from build123d import *

# Parameters (mm, degrees)
SKETCH28_W                                   = 80
SKETCH28_H                                   = 80
BOSS_EXTRUDE1_DEPTH                          = 10
CBORE_FOR_M10_CHEESE_HEAD_SCREW1_D           = 12
CBORE_FOR_M10_CHEESE_HEAD_SCREW1_CBORE_D     = 26
CBORE_FOR_M10_CHEESE_HEAD_SCREW1_CBORE_DEPTH = 5
SKETCH36_R                                   = 1
BOSS_EXTRUDE5_DEPTH                          = 10
SKETCH37_R                                   = 22.5
SKETCH37_R_2                                 = 15.5
CUT_EXTRUDE2_DEPTH                           = 6
CUT_EXTRUDE6_DEPTH                           = 6
SKETCH40_W                                   = 18.062589032
SKETCH40_H                                   = 3
BOSS_EXTRUDE7_DEPTH                          = 13


with BuildPart() as part:
    # Sketch28 → Boss-Extrude1 (new body)
    with BuildSketch(Plane(origin=(0, 0, 0), x_dir=(1, 0, 0), z_dir=(0, 1, 0))):
        with Locations((1.944585414, 4.241283073)):
            Rectangle(SKETCH28_W, SKETCH28_H)
    extrude(amount=BOSS_EXTRUDE1_DEPTH)

    # CBORE for M10 Cheese Head Screw1 (through all)
    with Locations(Plane(origin=(0, 10, 0), x_dir=(1, 0, 0), z_dir=(0, 1, 0))):
        with Locations((1.944585414, 4.241283073)):
            CounterBoreHole(CBORE_FOR_M10_CHEESE_HEAD_SCREW1_D / 2, CBORE_FOR_M10_CHEESE_HEAD_SCREW1_CBORE_D / 2, CBORE_FOR_M10_CHEESE_HEAD_SCREW1_CBORE_DEPTH)

    # Sketch36 → Boss-Extrude5 (add)
    with BuildSketch(Plane.XZ):
        with Locations(Location((12.444585414, -16.741283073, 0), (0, 0, 270))):
            Circle(SKETCH36_R)
        with Locations(Location((12.444585414, -4.241283073, 0), (0, 0, 270))):
            Circle(SKETCH36_R)
        with Locations(Location((-8.555414586, -16.741283073, 0), (0, 0, 90))):
            Circle(SKETCH36_R)
        with Locations(Location((-8.555414586, -4.241283073, 0), (0, 0, 90))):
            Circle(SKETCH36_R)
    extrude(amount=BOSS_EXTRUDE5_DEPTH)

    # Sketch37 → Cut-Extrude2 (cut)
    with BuildSketch(Plane(origin=(0, 10, 0), x_dir=(1, 0, 0), z_dir=(0, 1, 0))):
        with Locations(Location((1.944585414, 4.241283073, 0), (0, 0, 270))):
            Circle(SKETCH37_R)
        with Locations(Location((1.944585414, 4.241283073, 0), (0, 0, 270))):
            Circle(SKETCH37_R_2, mode=Mode.SUBTRACT)
    extrude(amount=-CUT_EXTRUDE2_DEPTH, mode=Mode.SUBTRACT)

    # Sketch39 → Cut-Extrude6 (cut)
    with BuildSketch(Plane(origin=(0, 10, 0), x_dir=(1, 0, 0), z_dir=(0, 1, 0))):
        with BuildLine():
            Line((6.944585414, -35.758716927), (6.944585414, -17.696127895))
            ThreePointArc((6.944585414, -17.696127895), (1.944585414, -18.258716927), (-3.055414586, -17.696127895))
            Line((-3.055414586, -17.696127895), (-3.055414586, -35.758716927))
            Line((-3.055414586, -35.758716927), (1.944585414, -35.758716927))
            Line((1.944585414, -35.758716927), (6.944585414, -35.758716927))
        make_face()
    extrude(amount=-CUT_EXTRUDE6_DEPTH, mode=Mode.SUBTRACT)

    # Sketch40 → Boss-Extrude7 (add)
    with BuildSketch(Plane(origin=(-3.055414586, 0, 0), x_dir=(0, 0, -1), z_dir=(1, 0, 0))):
        with Locations((-26.727422411, 8.5)):
            Rectangle(SKETCH40_W, SKETCH40_H)
    extrude(amount=BOSS_EXTRUDE7_DEPTH)


solid = part.part
Geometry check sheet. Reference: the model listing, model coordinates, mm. A direction names the side the tool comes from. Coordinates: 2 decimals unless noted, no trailing zeros. Order: outer loops, then holes, each group sorted by start corner. A loop starts at its lowest first (then second) coordinate and runs counter-clockwise, first axis right, second up. Notation, with made-up numbers: (30, 8) -> (61, 8) arc R19 ccw to (61, 25) -> close; hole circle Ø8 at (-1.75, 9.5). An arc over 180 degrees is marked (long way). Use a Markdown table: item, result. Add a question column.
1. Cross-section at A-A (z = 0). Enter the section's corners in (x, y).
2. Go/stop test with flat-tipped pins: pin 1 Ø24 at (x, z) = (12, 14.5) entering from -Y; pin 2 Ø13 at (x, z) = (5, -5) entering from +Y; pin 3 Ø23.5 at (x, z) = (1.94, -4.24) entering from -Y. Record where each tip stops, or that it passes through.
3. Cross-section at D-D (y = -4.25). Enter the section's corners in (x, z).
4. Mould release check, pull along X, two halves, no side actions. Record for faces 1 (the face through (2.863, 7.042, -26.723)), 2 (the face through (7.94, 2.46, -4.51)), 3 (the face through (-9, -10, -17)), 4 (the face through (-38.055, 5, -4)): pulls with the +X half, pulls with the -X half, needs draft (parallel to the pull), parting line crosses it, or undercut.
5. Set-up check for faces 5 (the face through (1, 5, -44.241)), 6 (the face through (11.557, -4.93, -4.703)), 7 (the face through (-0.87, 7.54, 8.45)), 8 (the face through (-16, 10, -21)), 9 (the face through (2, 7, 27)): record each of +Z, -Z, +X, -X, +Y, -Y from which the full face is reachable in a straight line by a thin tool's end or side.
6. Cross-section at B-B (z = 27). Enter the section's corners in (x, y).
7. Cross-section at C-C (x = -24). Enter the section's corners in (y, z), and give its area (3 significant figures).
8. Material ranges on L1, parallel to X at y = 5, z = 26; L2, parallel to Z at x = 10, y = 4.5; L3, parallel to X at y = 8.75, z = -12.5, recorded low to high.
Filled sheet:
| question | item | result |
|---|---|---|
| 1 | outline | (-38.06, 0) -> (-2.3, 0) -> (-2.3, 5) -> (-10.34, 5) -> (-10.34, 10) -> (-12.96, 10) -> (-12.96, 4) -> (-20.15, 4) -> (-20.15, 10) -> (-38.06, 10) -> close; (6.19, 0) -> (41.94, 0) -> (41.94, 10) -> (24.04, 10) -> (24.04, 4) -> (16.85, 4) -> (16.85, 10) -> (14.23, 10) -> (14.23, 5) -> (6.19, 5) -> close |
| 2 | pin 1 | y = 0 |
| 2 | pin 2 | y = 5 |
| 2 | pin 3 | y = -10 |
| 3 | outline | circle Ø2 at (-8.56, -16.74); circle Ø2 at (-8.56, -4.24); circle Ø2 at (12.44, -16.74); circle Ø2 at (12.44, -4.24) |
| 4 | face 1 | undercut |
| 4 | face 2 | undercut |
| 4 | face 3 | needs draft |
| 4 | face 4 | pulls with the -X half |
| 5 | face 5 | -Z, +X, -X, +Y, -Y |
| 5 | face 6 | -Y |
| 5 | face 7 | +Y |
| 5 | face 8 | +Z, -Z, +X, -X, +Y |
| 5 | face 9 | +Z |
| 6 | outline | (-38.06, 0) -> (41.94, 0) -> (41.94, 10) -> (-38.06, 10) -> close; hole (-3.06, 4) -> (6.94, 4) -> (6.94, 7) -> (-3.06, 7) -> close |
| 7 | outline | (0, -44.24) -> (10, -44.24) -> (10, 35.76) -> (0, 35.76) -> close |
| 7 | area | 800 mm2 |
| 8 | L1 | -38.06 to -3.06, 6.94 to 41.94 |
| 8 | L2 | -44.24 to -25.25, -17.48 to 9, 16.77 to 35.76 |
| 8 | L3 | -38.06 to -18.98, -11.17 to -8.1, 11.98 to 15.06, 22.87 to 41.94 |
